from build123d import *

# Parameters (mm, degrees)
SKETCH_2_R                   = 1.6
EXTRUDE_1_DEPTH              = 1.5
CUT_EXTRUDE_1_DEPTH          = 3
FILLET_1_R                   = 1
FILLET_2_R                   = 1.75
HOLE_WIZARD_M3_1_D           = 3.4
HOLE_WIZARD_M3_1_DEPTH       = 18.978536948
HOLE_WIZARD_M3_1_CSINK_D     = 6.3
HOLE_WIZARD_M3_1_CSINK_ANGLE = 90
HOLE_WIZARD_M3_1_TIP         = 1.021463052
MOVE_START                   = -1.5
MOVE_FACE_1_DEPTH            = 3


# Read off the part's stored shape, not the designer's step: 面の移動1
with BuildPart() as part:
    # ｽｹｯﾁ2 → ﾎﾞｽ - 押し出し1 (new, symmetric)
    with BuildSketch(Plane(origin=(0, 0, 0), x_dir=(1, 0, 0), z_dir=(0, 1, 0))):
        Polygon((24.47, 8.660254038), (9.47, 0), (0, 0), (0, -15), (30, -15), (55.450762114, 15), (50.450762114, 23.660254038), align=None)
        with Locations(Location((48.620635095, 16.830127019, 0), (0, 0, 270))):
            Circle(SKETCH_2_R, mode=Mode.SUBTRACT)
        with Locations(Location((25, -7.5, 0), (0, 0, 270))):
            Circle(SKETCH_2_R, mode=Mode.SUBTRACT)
        with Locations(Location((31.300127019, 6.830127019, 0), (0, 0, 270))):
            Circle(SKETCH_2_R, mode=Mode.SUBTRACT)
        with Locations(Location((5, -7.5, 0), (0, 0, 270))):
            Circle(SKETCH_2_R, mode=Mode.SUBTRACT)
    extrude(amount=EXTRUDE_1_DEPTH, both=True)

    # ｽｹｯﾁ3 → ｶｯﾄ - 押し出し1 (cut)
    with BuildSketch(Plane(origin=(0, 1.5, 0), x_dir=(1, 0, 0), z_dir=(0, 1, 0))):
        Polygon((26.47, 5.196152423), (17.47, 0), (27.140628594, 0), (27.879009742, 2.755675961), align=None)
        Polygon((33.352285677, 0), (37.479868618, 0), (45.169472556, 9.064094706), (34.062793268, 2.651650429), align=None)
        Polygon((31.44676478, -7.111500799), (37.479868618, 0), (33.352285677, 0), align=None)
    extrude(amount=-CUT_EXTRUDE_1_DEPTH, mode=Mode.SUBTRACT)

    # ﾌｨﾚｯﾄ1
    fillet_1_edges = [part.edges().sort_by_distance(p)[0] for p in [
        (27.879009742, 0, -2.755675961),
        (27.140628594, 0, 0),
        (17.47, 0, 0),
        (26.47, 0, -5.196152423),
        (34.062793268, 0, -2.651650429),
        (45.169472556, 0, -9.064094706),
        (31.44676478, 0, 7.111500799),
    ]]
    fillet(fillet_1_edges, radius=FILLET_1_R)

    # ﾌｨﾚｯﾄ2
    fillet_2_edges = [part.edges().sort_by_distance(p)[0] for p in [
        (50.450762114, 0, -23.660254038),
        (55.450762114, 0, -15),
        (30, 0, 15),
        (0, 0, 15),
        (0, 0, 0),
        (9.47, 0, 0),
    ]]
    fillet(fillet_2_edges, radius=FILLET_2_R)

    # M3 丸皿ねじ用皿穴1
    with Locations(Plane(origin=(5, 1.5, 7.5), x_dir=(0, 0, 1), z_dir=(0, 1, 0))):
        with Locations((0, 0), (0, 20), (-14.330127019, 26.300127019), (-24.330127019, 43.620635095)):
            CounterSinkHole(HOLE_WIZARD_M3_1_D / 2, HOLE_WIZARD_M3_1_CSINK_D / 2, depth=HOLE_WIZARD_M3_1_DEPTH, counter_sink_angle=HOLE_WIZARD_M3_1_CSINK_ANGLE)
            with Locations((0, 0, -(HOLE_WIZARD_M3_1_DEPTH + HOLE_WIZARD_M3_1_TIP / 2))):  # 118° drill point
                Cone(0, HOLE_WIZARD_M3_1_D / 2, HOLE_WIZARD_M3_1_TIP, mode=Mode.SUBTRACT)

    # Move Face 1 outline → Move Face 1 (cut)
    # profile 1 of 2: a face of its own
    with BuildSketch(Plane(origin=(0, 0, 0), x_dir=(1, 0, 0), z_dir=(0, 1, 0)).offset(MOVE_START)):
        with BuildLine():
            Line((39.92911769, 6.615924683), (34.171512735, 3.291769913))
            ThreePointArc((34.171512735, 3.291769913), (33.731482725, 2.90587395), (33.472623996, 2.380960375))
            Line((33.472623996, 2.380960375), (32.116497814, -2.680171439))
            ThreePointArc((32.116497814, -2.680171439), (32.869167953, -4.39703828), (34.709221416, -4.038782306))
            Line((34.709221416, -4.038782306), (41.822952552, 4.346504278))
            ThreePointArc((41.822952552, 4.346504278), (41.830787659, 6.27795696), (39.92911769, 6.615924683))
        make_face()
        with BuildLine():
            ThreePointArc((33.955586909, 2.251550852), (34.128159395, 2.601493236), (34.421512735, 2.858757211))
            Line((34.421512735, 2.858757211), (40.17911769, 6.182911981))
            ThreePointArc((40.17911769, 6.182911981), (41.44689767, 5.957600166), (41.441674265, 4.669965044))
            Line((41.441674265, 4.669965044), (34.327943128, -3.71532154))
            ThreePointArc((34.327943128, -3.71532154), (33.10124082, -3.954158856), (32.599460727, -2.809580962))
            Line((32.599460727, -2.809580962), (33.955586909, 2.251550852))
        make_face(mode=Mode.SUBTRACT)
    # profile 2 of 2: a face of its own
    with BuildSketch(Plane(origin=(0, 0, 0), x_dir=(1, 0, 0), z_dir=(0, 1, 0)).offset(MOVE_START)):
        with BuildLine():
            Line((27.822190346, 0.611771432), (28.254766297, 2.226166861))
            ThreePointArc((28.254766297, 2.226166861), (28.293044849, 2.810184717), (28.104915663, 3.364395428))
            Line((28.104915663, 3.364395428), (27.403012702, 4.580127019))
            ThreePointArc((27.403012702, 4.580127019), (26.492203164, 5.279015758), (25.353974596, 5.129165125))
            Line((25.353974596, 5.129165125), (20.452050808, 2.299038106))
            ThreePointArc((20.452050808, 2.299038106), (19.753162068, 0.611771432), (21.202050808, -0.5))
            Line((21.202050808, -0.5), (26.373301606, -0.5))
            ThreePointArc((26.373301606, -0.5), (27.286443749, -0.19003001), (27.822190346, 0.611771432))
        make_face()
        with BuildLine():
            Line((26.373301606, 0), (21.202050808, 0))
            ThreePointArc((21.202050808, 0), (20.236124981, 0.741180955), (20.702050808, 1.866025404))
            Line((20.702050808, 1.866025404), (25.603974596, 4.696152423))
            ThreePointArc((25.603974596, 4.696152423), (26.362793641, 4.796052845), (26.97, 4.330127019))
            Line((26.97, 4.330127019), (27.671902961, 3.114395428))
            ThreePointArc((27.671902961, 3.114395428), (27.797322419, 2.74492162), (27.771803384, 2.355576383))
            Line((27.771803384, 2.355576383), (27.339227432, 0.741180955))
            ThreePointArc((27.339227432, 0.741180955), (26.982063035, 0.20664666), (26.373301606, 0))
        make_face(mode=Mode.SUBTRACT)
    extrude(amount=MOVE_FACE_1_DEPTH, mode=Mode.SUBTRACT)


solid = part.part
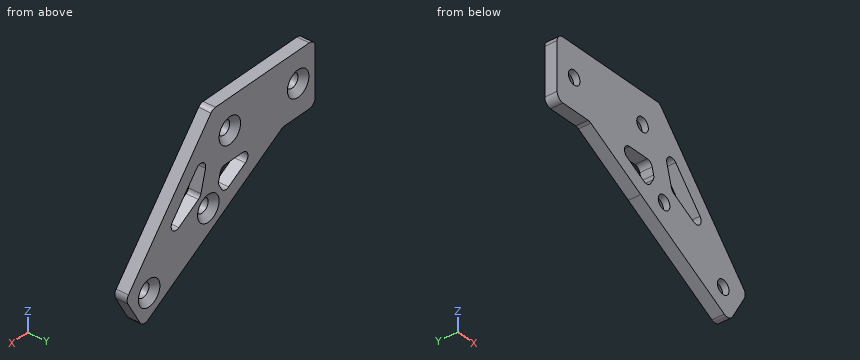
CAD build for the part. Positions are in the model's coordinates, mm. Coordinates: 2 decimals unless noted, no trailing zeros. Write each loop counter-clockwise with the first axis right and the second up, starting at its lowest first coordinate (ties: lowest second). Pieces come first, ordered by that corner, then holes. Notation, with made-up numbers: (-8, 37) - (22, 37) arc R16 cw to (22, 47) - close; hole circle Ø6 at (-18, 13.25). An arc over 180 degrees is marked (long way). Use a Markdown table: item, result. Add a question column.
Item 1: Band-saw the part on A-A, the plane x = 5. Give the cut face in (y, z).
Item 2: Band-saw the part on C-C, the plane z = 7.5. Give the cut face in (x, y), and give its area (3 significant figures).
Item 3: Band-saw the part on B-B, the plane y = 0.8. Give the number of separate pieces and of enclosed holes in the cut face, and give its area (3 significant figures).
Item 4: Flat gauge pins, fed straight in: pin 1 (4.5 mm diameter, centred on x = 25, z = 7.5, fed in from +Y); pin 2 (2 mm diameter, centred on x = 5, z = 7.5, fed in from +Y); pin 3 (1.5 mm diameter, centred on x = 5, y = 0, fed in from -Z); pin 4 (4 mm diameter, centred on x = 48.62, z = -16.83, fed in from +Y). Where does each tip first touch, or does it go through?
Item 5: Band-saw the part on D-D, the plane x = 36.5. Give the cut face in (y, z).
Item 6: Drill centre lines: L1, parallel to X at y = -0.25, z = 7.5; L2, parallel to Z at x = 5, y = -0.35; L3, parallel to Z at x = 25, y = -0.55. Where is each one in solid material? Low to high. Write a range as from..to.
Numbers:
| question | item | result |
|---|---|---|
| 1 | outline | (-1.5, 0) - (1.5, 0) - (1.5, 4.35) - (0.05, 5.8) - (-1.5, 5.8) - close; (-1.5, 9.2) - (0.05, 9.2) - (1.5, 10.65) - (1.5, 15) - (-1.5, 15) - close |
| 2 | outline | (0, -1.5) - (3.3, -1.5) - (3.3, 0.05) - (1.85, 1.5) - (0, 1.5) - close; (6.7, -1.5) - (23.3, -1.5) - (23.3, 0.05) - (21.85, 1.5) - (8.15, 1.5) - (6.7, 0.05) - close; (26.7, -1.5) - (36.36, -1.5) - (36.36, 1.5) - (28.15, 1.5) - (26.7, 0.05) - close |
| 2 | area | 84.5 mm2 |
| 3 | separate pieces | 1 |
| 3 | enclosed holes | 6 |
| 3 | area | 864 mm2 |
| 4 | pin 1 | y = 0.6 |
| 4 | pin 2 | through |
| 4 | pin 3 | z = 0 |
| 4 | pin 4 | y = 0.35 |
| 5 | outline | (-1.5, -15.61) - (1.5, -15.61) - (1.5, -4.64) - (-1.5, -4.64) - close; (-1.5, 1.93) - (1.5, 1.93) - (1.5, 7.34) - (-1.5, 7.34) - close |
| 6 | L1 | 0..3.3, 6.7..23.3, 26.7..36.36 |
| 6 | L2 | 0..5.8, 9.2..15 |
| 6 | L3 | -8.97..-4.92, 0.5..5.8, 9.2..15 |
